from build123d import *

# Parameters (mm, degrees)
SKETCH2_W          = 3
SKETCH2_H          = 10
CUT_EXTRUDE3_DEPTH = 5


with BuildPart() as part:
    # Sketch1 → Revolve1 (revolve)
    with BuildSketch(Plane.XY, mode=Mode.PRIVATE) as revolve1_sk:
        Polygon((30, -27.855726757), (30, 51.144273243), (40, 51.144273243), (40, 63.144273243), (47.5, 63.144273243), (47.5, 45.144273243), (42, 45.144273243), (42, 29.144273243), (40, 29.144273243), (40, -15.855726757), (42, -15.855726757), (42, -27.855726757), align=None)
    revolve(revolve1_sk.sketch.rotate(Axis((0, -44.504269507, 0), (0, 1, 0)), 90), axis=Axis((0, -44.504269507, 0), (0, 1, 0)))

    # Sketch2 → Cut-Extrude3 (cut, symmetric)
    with BuildSketch(Plane.XY):
        with Locations((-40.5, 40.144273243)):
            Rectangle(SKETCH2_W, SKETCH2_H)
    extrude(amount=CUT_EXTRUDE3_DEPTH, both=True, mode=Mode.SUBTRACT)


solid = part.part
Read the model definition and answer for the solid it produces. Units are mm, in the model's axes. A direction names the side the tool comes from. Coordinates: 2 decimals unless noted, no trailing zeros. Write each loop counter-clockwise with the first axis right and the second up, starting at its lowest first coordinate (ties: lowest second). Pieces come first, ordered by that corner, then holes. Notation, with made-up numbers: (-19, 19.25) - (6, 19.25) arc R21 cw to (6, 38.25) - close; hole circle Ø2 at (47, 25.5). An arc over 180 degrees is marked (long way). One line per question, with ' | ' between items.
Q1. Find section A-A, the plane z = 0. Write down the section's boundary in (x, y).
Result set:
outline: (-47.5, 45.14) - (-39, 45.14) - (-39, 35.14) - (-42, 35.14) - (-42, 29.14) - (-40, 29.14) - (-40, -15.86) - (-42, -15.86) - (-42, -27.86) - (-30, -27.86) - (-30, 51.14) - (-40, 51.14) - (-40, 63.14) - (-47.5, 63.14) - close; (30, -27.86) - (42, -27.86) - (42, -15.86) - (40, -15.86) - (40, 29.14) - (42, 29.14) - (42, 45.14) - (47.5, 45.14) - (47.5, 63.14) - (40, 63.14) - (40, 51.14) - (30, 51.14) - close
Q2. Find section B-B, the plane x = 0. Write down the section's boundary in (y, z), plus the area to 3 significant figures.
Result set:
outline: (-27.86, -42) - (-15.86, -42) - (-15.86, -40) - (29.14, -40) - (29.14, -42) - (45.14, -42) - (45.14, -47.5) - (63.14, -47.5) - (63.14, -40) - (51.14, -40) - (51.14, -30) - (-27.86, -30) - close; (-27.86, 30) - (51.14, 30) - (51.14, 40) - (63.14, 40) - (63.14, 47.5) - (45.14, 47.5) - (45.14, 42) - (29.14, 42) - (29.14, 40) - (-15.86, 40) - (-15.86, 42) - (-27.86, 42) - close | area: 1,960 mm^2
Q3. Find section C-C, the plane y = 20. Write down the section's boundary in (x, z), plus the area to 3 significant figures.
Result set:
outline: circle Ø80 at (0, 0); hole circle Ø60 at (0, 0) | area: 2,200 mm^2
Q4. Each of these flat-tipped pins is pushed along its axis until it touches: P1, Ø10, axis at y = 30.5, z = 0.5, coming from the -X side; P2, Ø1, axis at x = 5, z = 33.5, coming from the +Y side; P3, Ø3, axis at y = 38, z = 2, coming from the -X side. Where does it stop, or does it pass through?
Result set:
P1: x = -42 | P2: y = 51.14 | P3: x = -39
Q5. Determine the mould class of faces 1 (the flat face through (15.4, 29.144, -37.1)), 2 (the cylindrical face through (-1.76, 57.23, 39.96)), 3 (the flat face through (35, 63.144, -21)) for opening direction Y: +Y half, -Y half, draft (parallel to the pull), parting line (faces both ways), or undercut.
Result set:
face 1: undercut | face 2: draft | face 3: +Y half
Q6. For faces 4 (the cylindrical face through (-12.62, 37.03, -40.06)), 5 (the flat face through (15.4, -15.856, 37.1)), 6 (the flat face through (-30, 51.144, 6)), determine the directions among +Z, -Z, +X, -X, +Y, -Y from which every point of the face is accessible in a straight line to the end or side of a thin tool.
Result set:
face 4: -Y | face 5: none | face 6: +Y
Q7. Consider L1, parallel to Y at x = -38, z = 15; L2, parallel to X at y = 58.5, z = 0; L3, parallel to Y at x = 34.5, z = -25.5. Determine where each line is inside the solid, lowest interval first. Write a range as [from, to].
Result set:
L1: [-27.86, -15.86], [29.14, 63.14] | L2: [-47.5, -40], [40, 47.5] | L3: [45.14, 63.14]
Q8. Find section D-D, the plane z = 35. Write down the section's boundary in (x, y), plus the area to 3 significant figures.
Result set:
outline: (-32.11, 45.14) - (-23.22, 45.14) - (-23.22, 29.14) - (-19.36, 29.14) - (-19.36, -15.86) - (-23.22, -15.86) - (-23.22, -27.86) - (23.22, -27.86) - (23.22, -15.86) - (19.36, -15.86) - (19.36, 29.14) - (23.22, 29.14) - (23.22, 45.14) - (32.11, 45.14) - (32.11, 63.14) - (19.36, 63.14) - (19.36, 51.14) - (-19.36, 51.14) - (-19.36, 63.14) - (-32.11, 63.14) - close | area: 3,730 mm^2
